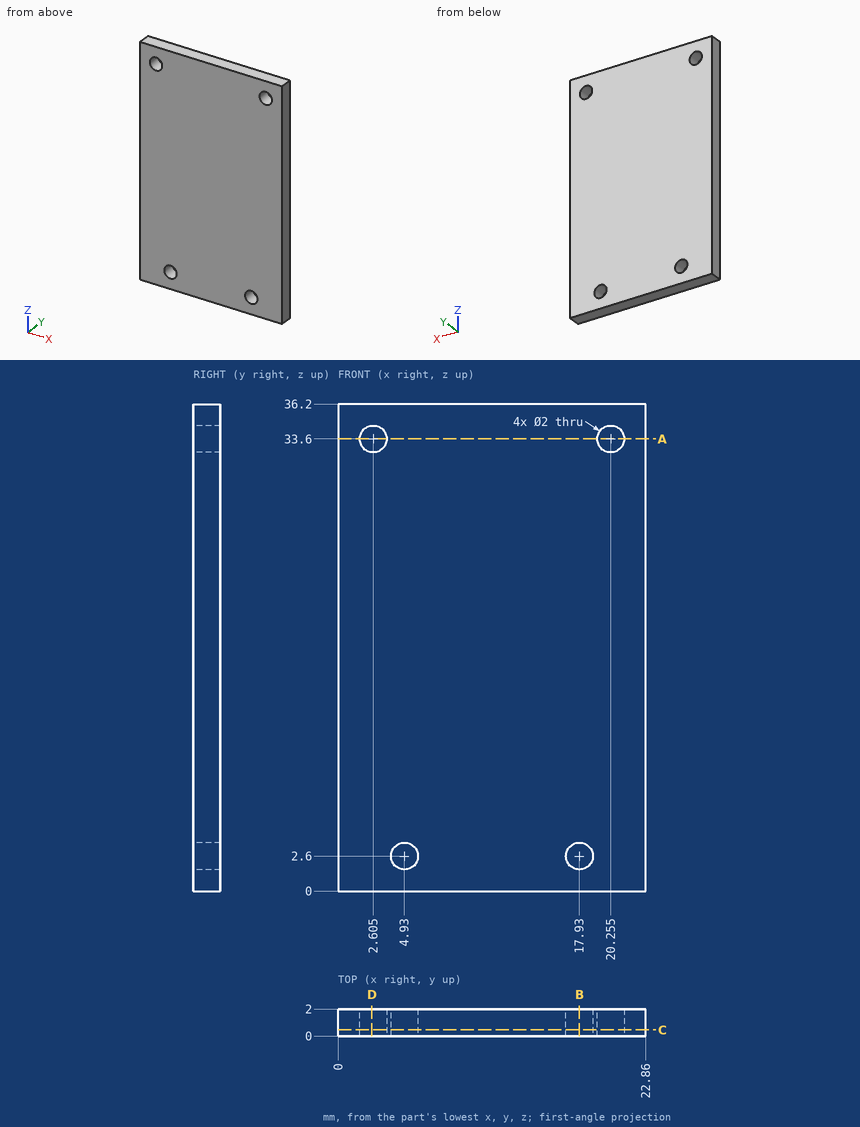
Geometry: see drawing. Coordinates: mm, zero at the bounding-box minimum. Give positions to 0.01 mm unless a question says otherwise; leave off trailing zeros. Write each loop counter-clockwise with the first axis right and the second up, starting at its lowest first coordinate (ties: lowest second). Pieces come first, ordered by that corner, then holes. Notation, with made-up numbers: M 12,-36 L 25,-36 A6 ccw 25,-25 Z; hole C 36,84 d2. An arc over 180 degrees is marked long. Return JSON: item names as keys, results as strings. Group by question number.
1) Cut plane A-A, the plane z = 33.6. Output: boundary loops of the cut face in (x, y) (3 decimals).
2) Cut plane C-C, the plane y = 0.45. Output: boundary loops of the cut face in (x, z) (3 decimals), then the cut area to 3 significant figures.
3) Cut plane B-B, the plane x = 17.93. Output: boundary loops of the cut face in (y, z), then the cut area to 3 significant figures.
4) Cut plane D-D, the plane x = 2.5. Output: boundary loops of the cut face in (y, z).
5) Ray query, L1, parallel to Z at x = 4.93, y = 1.4; L2, parallel to Z at x = 2.5, y = 1.45; L3, parallel to X at y = 0.2, z = 33 (3 decimals). Return the intervals inside material, ascending.
Data:
{
 "1": {"outline": "M 0,0 L 1.605,0 L 1.605,2 L 0,2 Z; M 3.605,0 L 19.255,0 L 19.255,2 L 3.605,2 Z; M 21.255,0 L 22.86,0 L 22.86,2 L 21.255,2 Z"},
 "2": {"outline": "M 0,0 L 22.86,0 L 22.86,36.2 L 0,36.2 Z; hole C 2.605,33.6 d2; hole C 4.93,2.6 d2; hole C 17.93,2.6 d2; hole C 20.255,33.6 d2", "area": "815 mm²"},
 "3": {"outline": "M 0,0 L 2,0 L 2,1.6 L 0,1.6 Z; M 0,3.6 L 2,3.6 L 2,36.2 L 0,36.2 Z", "area": "68.4 mm²"},
 "4": {"outline": "M 0,0 L 2,0 L 2,32.61 L 0,32.61 Z; M 0,34.59 L 2,34.59 L 2,36.2 L 0,36.2 Z"},
 "5": {"L1": "z = 0 to 1.6, 3.6 to 36.2", "L2": "z = 0 to 32.61, 34.59 to 36.2", "L3": "x = 0 to 1.805, 3.405 to 19.455, 21.055 to 22.86"}
}
